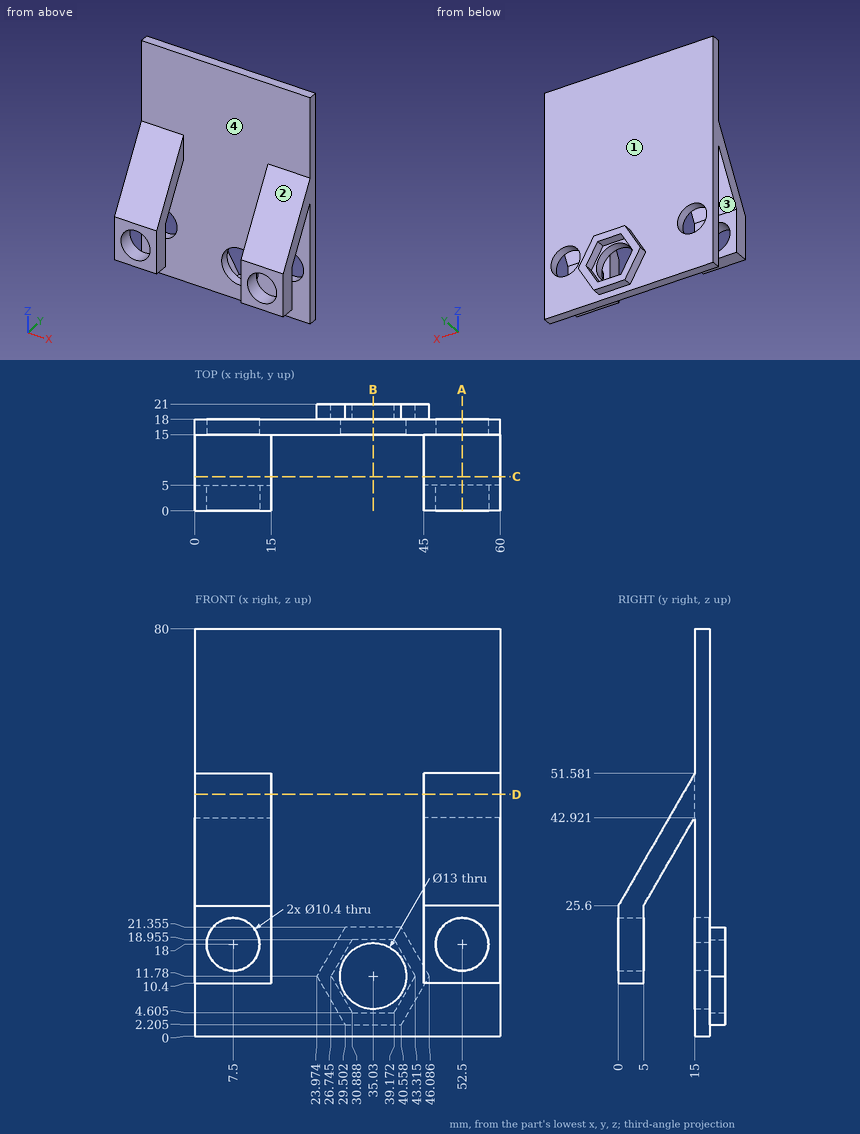
The drawing under review shows one solid part. Ordinate dimensions are in mm from its lowest x, y, z. Coordinates: 2 decimals unless noted, no trailing zeros. Order: outer loops, then holes, each group sorted by start corner. A loop starts at its lowest first (then second) coordinate and runs counter-clockwise, first axis right, second up. Notation, with made-up numbers: (-7, -12.75) -> (15, -12.75) arc R24 ccw to (15, 0.25) -> close; hole circle Ø11 at (75, 83.25). An arc over 180 degrees is marked (long way). Return JSON: item names as keys, results as strings.
1. For pin 1 Ø6 at (x, z) = (52.5, 18) entering from +Y; pin 2 Ø2.5 at (x, y) = (10.5, 3.5) entering from -Z; pin 3 Ø16.5 at (x, z) = (53.5, 21) entering from +Y; pin 4 Ø2.5 at (x, y) = (33.5, 20) entering from -Z (1 decimal), all flat-tipped, find the tip position at first contact; note any pin that passes through.
Answer block:
{"pin 1": "through", "pin 2": "z = 10.4", "pin 3": "y = 18", "pin 4": "z = 2.2"}
2. We need section D-D on z = 47.5. Write out the cut boundary in (x, y), and give its area (3 significant figures).
Answer block:
{"outline": "(0, 12.64) -> (15, 12.64) -> (15, 15) -> (45, 15) -> (45, 12.64) -> (60, 12.64) -> (60, 18) -> (0, 18) -> close", "area": "251 mm²"}
3. We need section A-A on x = 52.5. Write out the cut boundary in (y, z).
Answer block:
{"outline": "(0, 10.4) -> (5, 10.4) -> (5, 12.8) -> (0, 12.8) -> close; (0, 23.2) -> (5, 23.2) -> (5, 25.6) -> (15, 42.92) -> (15, 23.2) -> (18, 23.2) -> (18, 80) -> (15, 80) -> (15, 51.58) -> (0, 25.6) -> close; (15, 0) -> (18, 0) -> (18, 12.8) -> (15, 12.8) -> close"}
4. We need section C-C on y = 6.75. Write out the cut boundary in (x, z), and give its area (3 significant figures).
Answer block:
{"outline": "(0, 28.63) -> (15, 28.63) -> (15, 37.29) -> (0, 37.29) -> close; (45, 28.63) -> (60, 28.63) -> (60, 37.29) -> (45, 37.29) -> close", "area": "260 mm²"}
5. The part is to be moulded in two halves that separate along Y. For the marked faces 1, 2, 3 and 4, say which applies: +Y half, -Y half, draft (parallel to the pull), parting line (faces both ways), or undercut.
Answer block:
{"face 1": "+Y half", "face 2": "-Y half", "face 3": "undercut", "face 4": "undercut"}
6. For line 1 (X direction, y = 2.4, z = 18); line 2 (Z direction, x = 35.03, y = 16.95); line 3 (Z direction, x = 7.5, y = 16.2), list the stretches that pass through material, from the lowest coordinate up. Write a range as from..to.
Answer block:
{"line 1": "0..2.3, 12.7..15, 45..47.3, 57.7..60", "line 2": "0..5.28, 18.28..80", "line 3": "0..12.8, 23.2..80"}
7. We need section B-B on x = 35.03. Write out the cut boundary in (y, z) (1 decimal).
Answer block:
{"outline": "(15, 0) -> (18, 0) -> (18, 2.2) -> (21, 2.2) -> (21, 4.6) -> (18, 4.6) -> (18, 5.3) -> (15, 5.3) -> close; (15, 18.3) -> (18, 18.3) -> (18, 19) -> (21, 19) -> (21, 21.4) -> (18, 21.4) -> (18, 80) -> (15, 80) -> close"}
